from build123d import *

# Parameters (mm, degrees)
SKETCH1_W                    = 496
SKETCH1_H                    = 520
BOSS_EXTRUDE1_DEPTH          = 4
EDGE_FLANGE1_STRIP_W         = 26
EDGE_FLANGE1_STRIP_H         = 4
EDGE_FLANGE1_STRIP_CUT_DEPTH = 520
EDGE_FLANGE1_DEPTH           = 520
EDGE_FLANGE2_STRIP_W         = 26
EDGE_FLANGE2_STRIP_H         = 4
EDGE_FLANGE2_STRIP_CUT_DEPTH = 520
EDGE_FLANGE2_DEPTH           = 520
CUT_EXTRUDE1_REACH           = 721.733
SKETCH17_R                   = 4
CUT_EXTRUDE2_REACH           = 721.733
SKETCH19_R                   = 4
BOSS_EXTRUDE2_DEPTH          = 35
SKETCH21_W                   = 100
SKETCH21_H                   = 6
BOSS_EXTRUDE3_DEPTH          = 10


# Sheet-metal steps are written as plain solids
with BuildPart() as part:
    # Sketch1 → Boss-Extrude1 (new body)
    with BuildSketch(Plane(origin=(0, 0, 0), x_dir=(1, 0, 0), z_dir=(0, 1, 0))):
        with Locations((248, 260)):
            Rectangle(SKETCH1_W, SKETCH1_H)
    extrude(amount=BOSS_EXTRUDE1_DEPTH)

    # Edge-Flange1 strip (across the edge) → Edge-Flange1 strip cut (cut)
    with BuildSketch(Plane(origin=(0, 4, -520), x_dir=(1, 0, 0), z_dir=(0, 0, 1))):
        with Locations((-4, -2)):
            Rectangle(EDGE_FLANGE1_STRIP_W, EDGE_FLANGE1_STRIP_H)
    extrude(amount=EDGE_FLANGE1_STRIP_CUT_DEPTH, mode=Mode.SUBTRACT)

    # Edge-Flange1 section (across the edge) → Edge-Flange1 (add)
    with BuildSketch(Plane(origin=(0, 4, -520), x_dir=(1, 0, 0), z_dir=(0, 0, 1))):
        with BuildLine():
            Line((0, 5), (0, 36))
            Line((0, 36), (4, 36))
            Line((4, 36), (4, 5))
            ThreePointArc((4, 5), (5.464466094, 1.464466094), (9, 0))
            Line((9, 0), (9, -4))
            ThreePointArc((9, -4), (2.636038969, -1.363961031), (0, 5))
        make_face()
    extrude(amount=EDGE_FLANGE1_DEPTH)

    # Edge-Flange2 strip (across the edge) → Edge-Flange2 strip cut (cut)
    with BuildSketch(Plane(origin=(496, 4, 0), x_dir=(-1, 0, 0), z_dir=(0, 0, -1))):
        with Locations((-4, -2)):
            Rectangle(EDGE_FLANGE2_STRIP_W, EDGE_FLANGE2_STRIP_H)
    extrude(amount=EDGE_FLANGE2_STRIP_CUT_DEPTH, mode=Mode.SUBTRACT)

    # Edge-Flange2 section (across the edge) → Edge-Flange2 (add)
    with BuildSketch(Plane(origin=(496, 4, 0), x_dir=(-1, 0, 0), z_dir=(0, 0, -1))):
        with BuildLine():
            Line((0, 5), (0, 36))
            Line((0, 36), (4, 36))
            Line((4, 36), (4, 5))
            ThreePointArc((4, 5), (5.464466094, 1.464466094), (9, 0))
            Line((9, 0), (9, -4))
            ThreePointArc((9, -4), (2.636038969, -1.363961031), (0, 5))
        make_face()
    extrude(amount=EDGE_FLANGE2_DEPTH)

    # Sketch17 → Cut-Extrude1 (cut, up to next)
    with BuildSketch(Plane.ZY, mode=Mode.PRIVATE) as cut_extrude1_sk1:
        with Locations(Location((-390, 20, 0), (0, 0, 270))):
            Circle(SKETCH17_R)
    cut_extrude1_tool1 = extrude(cut_extrude1_sk1.sketch, amount=-CUT_EXTRUDE1_REACH, mode=Mode.PRIVATE) & part.part
    # Sketch17 → Cut-Extrude1 (cut, up to next)
    with BuildSketch(Plane.ZY, mode=Mode.PRIVATE) as cut_extrude1_sk2:
        with Locations(Location((-260, 20, 0), (0, 0, 270))):
            Circle(SKETCH17_R)
    cut_extrude1_tool2 = extrude(cut_extrude1_sk2.sketch, amount=-CUT_EXTRUDE1_REACH, mode=Mode.PRIVATE) & part.part
    # Sketch17 → Cut-Extrude1 (cut, up to next)
    with BuildSketch(Plane.ZY, mode=Mode.PRIVATE) as cut_extrude1_sk3:
        with Locations(Location((-130, 20, 0), (0, 0, 270))):
            Circle(SKETCH17_R)
    cut_extrude1_tool3 = extrude(cut_extrude1_sk3.sketch, amount=-CUT_EXTRUDE1_REACH, mode=Mode.PRIVATE) & part.part
    add(cut_extrude1_tool1.solids().sort_by_distance((0, 20, -390))[0], mode=Mode.SUBTRACT)
    add(cut_extrude1_tool2.solids().sort_by_distance((0, 20, -260))[0], mode=Mode.SUBTRACT)
    add(cut_extrude1_tool3.solids().sort_by_distance((0, 20, -130))[0], mode=Mode.SUBTRACT)

    # Sketch19 → Cut-Extrude2 (cut, up to next)
    with BuildSketch(Plane(origin=(496, 0, 0), x_dir=(0, 0, -1), z_dir=(1, 0, 0)), mode=Mode.PRIVATE) as cut_extrude2_sk1:
        with Locations(Location((130, 20, 0), (0, 0, 270))):
            Circle(SKETCH19_R)
    cut_extrude2_tool1 = extrude(cut_extrude2_sk1.sketch, amount=-CUT_EXTRUDE2_REACH, mode=Mode.PRIVATE) & part.part
    # Sketch19 → Cut-Extrude2 (cut, up to next)
    with BuildSketch(Plane(origin=(496, 0, 0), x_dir=(0, 0, -1), z_dir=(1, 0, 0)), mode=Mode.PRIVATE) as cut_extrude2_sk2:
        with Locations(Location((260, 20, 0), (0, 0, 270))):
            Circle(SKETCH19_R)
    cut_extrude2_tool2 = extrude(cut_extrude2_sk2.sketch, amount=-CUT_EXTRUDE2_REACH, mode=Mode.PRIVATE) & part.part
    # Sketch19 → Cut-Extrude2 (cut, up to next)
    with BuildSketch(Plane(origin=(496, 0, 0), x_dir=(0, 0, -1), z_dir=(1, 0, 0)), mode=Mode.PRIVATE) as cut_extrude2_sk3:
        with Locations(Location((390, 20, 0), (0, 0, 270))):
            Circle(SKETCH19_R)
    cut_extrude2_tool3 = extrude(cut_extrude2_sk3.sketch, amount=-CUT_EXTRUDE2_REACH, mode=Mode.PRIVATE) & part.part
    add(cut_extrude2_tool1.solids().sort_by_distance((496, 20, -130))[0], mode=Mode.SUBTRACT)
    add(cut_extrude2_tool2.solids().sort_by_distance((496, 20, -260))[0], mode=Mode.SUBTRACT)
    add(cut_extrude2_tool3.solids().sort_by_distance((496, 20, -390))[0], mode=Mode.SUBTRACT)

    # Sketch20 → Boss-Extrude2 (add)
    with BuildSketch(Plane(origin=(0, 4, 0), x_dir=(1, 0, 0), z_dir=(0, 1, 0))):
        Polygon((34, 448.5), (74, 448.5), (74, 442.5), (40, 442.5), (40, 408.5), (34, 408.5), align=None)
        Polygon((234, 448.5), (194, 448.5), (194, 442.5), (228, 442.5), (228, 408.5), (234, 408.5), align=None)
        Polygon((234, 71.5), (194, 71.5), (194, 77.5), (228, 77.5), (228, 111.5), (234, 111.5), align=None)
        Polygon((34, 71.5), (34, 111.5), (40, 111.5), (40, 77.5), (74, 77.5), (74, 71.5), align=None)
        Polygon((262, 448.5), (302, 448.5), (302, 442.5), (268, 442.5), (268, 408.5), (262, 408.5), align=None)
        Polygon((462, 448.5), (422, 448.5), (422, 442.5), (456, 442.5), (456, 408.5), (462, 408.5), align=None)
        Polygon((262, 71.5), (302, 71.5), (302, 77.5), (268, 77.5), (268, 111.5), (262, 111.5), align=None)
        Polygon((462, 71.5), (462, 111.5), (456, 111.5), (456, 77.5), (422, 77.5), (422, 71.5), align=None)
    extrude(amount=BOSS_EXTRUDE2_DEPTH)

    # Sketch21 → Boss-Extrude3 (add)
    with BuildSketch(Plane(origin=(0, 4, 0), x_dir=(1, 0, 0), z_dir=(0, 1, 0))):
        with Locations((248, 28)):
            Rectangle(SKETCH21_W, SKETCH21_H)
        with Locations((248, 492)):
            Rectangle(SKETCH21_W, SKETCH21_H)
    extrude(amount=BOSS_EXTRUDE3_DEPTH)


solid = part.part
Could you check a few things on this model? Use its own coordinates, in mm. A direction names the side the tool comes from. Coordinates: 2 decimals unless noted, no trailing zeros. Order: outer loops, then holes, each group sorted by start corner. A loop starts at its lowest first (then second) coordinate and runs counter-clockwise, first axis right, second up.
Q1. Thinking about a two-plate mould opening in X: for faces 1 (the flat face through (282, 21, -71.5)), 2 (the flat face through (496, 24, -256)), which applies, released by +X, released by -X, zero draft, split by the parting line, or undercut?
Q2. Suppose I cut it at C-C on z = -305. Please give me the cut outline in (x, y).
Q3. Will these pins go through, and if not, where does the flat tip stop? pin 1 (6.5 mm diameter, centred on x = 231, y = 27, fed in from -Z); pin 2 (3 mm diameter, centred on x = 60.5, y = 29, fed in from +Z); pin 3 (2 mm diameter, centred on x = 257.5, z = -60, fed in from +Y).
Q4. Which directions (+Z, -Z, +X, -X, +Y, -Y) give clear straight access to the entire face, cutting with the end or side of a thin tool? Please do faces 3 (the flat face through (462, 21, -428)), 4 (the flat face through (268, 21, -426)), 5 (the flat face through (442, 21, -448.5)).
Q5. Suppose I cut it at A-A on z = -421. Please give me the cut outline in (x, y), and give its area (3 significant figures).
Q6. Please list where these lines run through material, in increasing order: L1, parallel to Z at x = 493, y = 20; L2, parallel to X at y = 10.5, z = -88.5; L3, parallel to X at y = 15.5, z = -32.
Q7. Suppose I cut it at B-B on x = 139. Please give me the cut outline in (y, z), and give its area (3 significant figures).
Answer:
1. face 1: undercut
1. face 2: released by +X
2. outline: (0, 9) arc R9 ccw to (9, 0) - (487, 0) arc R9 ccw to (496, 9) - (496, 40) - (492, 40) - (492, 9) arc R5 cw to (487, 4) - (9, 4) arc R5 cw to (4, 9) - (4, 40) - (0, 40) - close
3. pin 1: stops at z = -448.5
3. pin 2: stops at z = -71.5
3. pin 3: stops at y = 4
4. face 3: +Z, -Z, +Y
4. face 4: +Y
4. face 5: -Z, +Y
5. outline: (0, 9) arc R9 ccw to (9, 0) - (487, 0) arc R9 ccw to (496, 9) - (496, 40) - (492, 40) - (492, 9) arc R5 cw to (487, 4) - (462, 4) - (462, 39) - (456, 39) - (456, 4) - (268, 4) - (268, 39) - (262, 39) - (262, 4) - (234, 4) - (234, 39) - (228, 39) - (228, 4) - (40, 4) - (40, 39) - (34, 39) - (34, 4) - (9, 4) arc R5 cw to (4, 9) - (4, 40) - (0, 40) - close
5. area: 3,090 mm2
6. L1: z = -520 to -394, -386 to -264, -256 to -134, -126 to 0
6. L2: x = 0 to 4, 34 to 40, 228 to 234, 262 to 268, 456 to 462, 492 to 496
6. L3: x = 0 to 4, 492 to 496
7. outline: (0, -520) - (4, -520) - (4, 0) - (0, 0) - close
7. area: 2,080 mm2
